The listing builds one solid part. Answer for the finished solid, in the listing's coordinates (mm). A direction names the side the tool comes from. Coordinates: 2 decimals unless noted, no trailing zeros. Write each loop counter-clockwise with the first axis right and the second up, starting at its lowest first coordinate (ties: lowest second). Pieces come first, ordered by that corner, then holes.
from build123d import *

# Parameters (mm, degrees)
BOSS_EXTRUDE1_DEPTH = 3.175
CUT_EXTRUDE2_START  = 3.175
SKETCH2_R           = 5.1562
CUT_EXTRUDE2_DEPTH  = 116.03462534
CUT_EXTRUDE4_START  = 3.175
SKETCH3_R           = 1.89865
CUT_EXTRUDE4_DEPTH  = 12.7


with BuildPart() as part:
    # Sketch1 → Boss-Extrude1 (new, symmetric)
    with BuildSketch(Plane(origin=(0, 0, 0), x_dir=(1, 0, 0), z_dir=(0, 1, 0))):
        Polygon((-87.3125, -69.85), (87.3125, -69.85), (87.3125, 19.05), (23.8125, 19.05), (23.8125, 44.45), (-39.6875, 44.45), (-39.6875, 69.85), (-87.3125, 69.85), align=None)
    extrude(amount=BOSS_EXTRUDE1_DEPTH, both=True)

    # Sketch2 → Cut-Extrude2 (cut, through all)
    with BuildSketch(Plane(origin=(0, 0, 0), x_dir=(1, 0, 0), z_dir=(0, 1, 0)).offset(CUT_EXTRUDE2_START)):
        with Locations(Location((-30.1625, 0, 0), (0, 0, 270))):
            Circle(SKETCH2_R)
        with Locations(Location((33.3375, 0, 0), (0, 0, 270))):
            Circle(SKETCH2_R)
    extrude(amount=-CUT_EXTRUDE2_DEPTH, mode=Mode.SUBTRACT)

    # Sketch3 → Cut-Extrude4 (cut)
    with BuildSketch(Plane(origin=(0, 0, 0), x_dir=(1, 0, 0), z_dir=(0, 1, 0)).offset(CUT_EXTRUDE4_START)):
        with Locations(Location((-77.7875, 4.7752, 0), (0, 0, 270))):
            Circle(SKETCH3_R)
        with Locations(Location((-48.4251, 64.3128, 0), (0, 0, 270))):
            Circle(SKETCH3_R)
        with Locations(Location((-14.2875, -20.6248, 0), (0, 0, 270))):
            Circle(SKETCH3_R)
        with Locations(Location((15.0749, 38.9128, 0), (0, 0, 270))):
            Circle(SKETCH3_R)
        with Locations(Location((49.2125, -46.0248, 0), (0, 0, 270))):
            Circle(SKETCH3_R)
        with Locations(Location((78.5749, 13.5128, 0), (0, 0, 270))):
            Circle(SKETCH3_R)
    extrude(amount=-CUT_EXTRUDE4_DEPTH, mode=Mode.SUBTRACT)


solid = part.part
Q1. Given pin 1 (3 mm diameter, centred on y = -0.5, z = -31, fed in from +X); pin 2 (5 mm diameter, centred on x = -77.79, z = -4.78, fed in from +Y) (3 decimals); pin 3 (1.5 mm diameter, centred on x = -36, y = -0.5, fed in from -Z); pin 4 (1.9 mm diameter, centred on y = -1, z = -53, fed in from +X), each flat-ended and moving along its own axis, determine where each tip first touches the part or whether it passes through.
Answers below:
pin 1: stops at x = 23.81
pin 2: stops at y = 3.175
pin 3: stops at z = -44.45
pin 4: stops at x = -39.69
Q2. The part is cut by section D-D, the plane y = 0.25. State how many separate pieces and enclosed holes the cut face has, then the cut area to 3 significant figures.
Answers below:
separate pieces: 1
enclosed holes: 8
area: 19,300 mm2
Q3. Determine the mould class of faces 1 (the face through (56, 0, -19.05)), 2 (the face through (13.92, 0.04, -40.42)), 3 (the face through (76.89, 0.04, -12.64)), 4 (the face through (-39.688, 0, -57)) for opening direction X: released by +X, released by -X, zero draft, split by the parting line, or undercut.
Answers below:
face 1: zero draft
face 2: undercut
face 3: undercut
face 4: released by +X
Q4. The part is cut by section B-B, the plane z = 46. Write down the section's boundary in (x, y) (1 decimal).
Answers below:
outline: (-87.3, -3.2) - (47.3, -3.2) - (47.3, 3.2) - (-87.3, 3.2) - close; (51.1, -3.2) - (87.3, -3.2) - (87.3, 3.2) - (51.1, 3.2) - close
Q5. Which of the six approach directions +Z, -Z, +X, -X, +Y, -Y give full straight-line access (tool end or side, diameter ignored) to faces 5 (the face through (23.812, 0, -32)), 6 (the face through (-1, -3.175, 15))?
Answers below:
face 5: -Z, +X, +Y, -Y
face 6: +Z, -Z, +X, -X, -Y
Q6. The part is cut by section A-A, the plane z = 0. Write down the section's boundary in (x, y) (1 decimal).
Answers below:
outline: (-87.3, -3.2) - (-35.3, -3.2) - (-35.3, 3.2) - (-87.3, 3.2) - close; (-25, -3.2) - (28.2, -3.2) - (28.2, 3.2) - (-25, 3.2) - close; (38.5, -3.2) - (87.3, -3.2) - (87.3, 3.2) - (38.5, 3.2) - close
Q7. Find the intervals of material crossed by probe 1 along X at (y, z) = (-0.75, 0); probe 2 along Z at (x, y) = (46, 1.75); probe 3 along Z at (x, y) = (-37, -2), in increasing order.
Answers below:
probe 1: x = -87.31 to -35.32, -25.01 to 28.18, 38.49 to 87.31
probe 2: z = -19.05 to 69.85
probe 3: z = -44.45 to 69.85
Q8. The part is cut by section C-C, the plane x = 1. Write down the section's boundary in (y, z) (3 decimals), then the cut area to 3 significant figures.
Answers below:
outline: (-3.175, -44.45) - (3.175, -44.45) - (3.175, 69.85) - (-3.175, 69.85) - close
area: 726 mm2
